Build history of the part. All positions in model axes, mm. Face numbers are marked on the shaded views. Give positions to 0.01 mm unless a question says otherwise; leave off trailing zeros. Loops run counter-clockwise (first coordinate to the right, second up) from the corner with the lowest first, then second, coordinate; pieces in that order, holes last. Notation, with made-up numbers: M 54.25,19.25 L 77.25,19.25 A13 cw 77.25,31.25 Z; hole C 41.25,38.25 d7. An arc over 180 degrees is marked long. Answer as a JSON object with one key per item and string values. Group by question number.
1. Mould opens along X. For the marked faces 1, 2, 3 and 4 say: released by +X, released by -X, zero draft, split by the parting line, or undercut.
2. Slice it at A-A (x = 0). List the corners of the cut face in (y, z).
3. Drill centre lines: line 1 along Y through (x, z) = (0, 3.2); line 2 along Z through (x, y) = (-1, -2); line 3 along Z through (x, y) = (-12.25, 1.5). Where is each one in solid material? Low to high. Write a range as [from, to].
4. Slice it at B-B (z = 0.3). List the corners of the cut face in (x, y) (3 decimals), then the cut area to 3 significant figures.
5. Drop flat-ended pins along their axis: pin 1 Ø1.5 at (x, z) = (-10.5, 3.5) entering from -Y; pin 2 Ø2 at (y, z) = (2.5, 0.5) entering from -X; pin 3 Ø3 at (x, y) = (0, 0) entering from +Z; pin 4 Ø1.7 at (x, y) = (-6.5, -1) entering from +Z. Give the stop position or say it passes through.
6. Slice it at D-D (z = 2.25). List the corners of the cut face in (x, y) (3 decimals).
7. Slice it at C-C (y = 0). Give the number of separate pieces and of enclosed holes in the cut face, then the cut area to 3 significant figures.
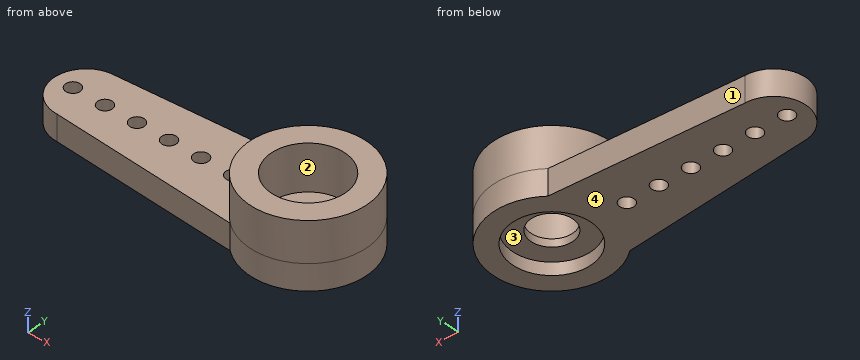
from build123d import *
from build123d.topology import SkipClean

# Parameters (mm, degrees)
RESSALTO_EXTRUS_O1_DEPTH = 1.6
ESBO_O2_R                = 3.65
RESSALTO_EXTRUS_O2_DEPTH = 2.5
ESBO_O3_R                = 2.3
CORTE_EXTRUS_O1_DEPTH    = 2.84
CORTE_EXTRUS_O2_REACH    = 18.456
ESBO_O4_R                = 0.45
ESBO_O5_R                = 1.3
CORTE_EXTRUS_O3_DEPTH    = 2.84
ESBO_O6_R                = 2.45
CORTE_EXTRUS_O4_DEPTH    = 0.78


with BuildPart() as part:
    # Esboço1 → Ressalto-extrusão1 (new body)
    with BuildSketch(Plane.XY):
        with BuildLine():
            Line((-13.85, 2), (-2.311249662, 2.825))
            ThreePointArc((-2.311249662, 2.825), (3.65, 0), (-2.311249662, -2.825))
            Line((-2.311249662, -2.825), (-13.85, -2))
            ThreePointArc((-13.85, -2), (-15.85, 0), (-13.85, 2))
        make_face()
    extrude(amount=RESSALTO_EXTRUS_O1_DEPTH)

    # Esboço2 → Ressalto-extrusão2 (add)
    with SkipClean():  # the faces are left unmerged after this step: merging them gives an invalid solid
        with BuildSketch(Plane.XY.offset(1.6)):
            with Locations(Location((0, 0, 0), (0, 0, 230.711977832))):
                Circle(ESBO_O2_R)
        extrude(amount=RESSALTO_EXTRUS_O2_DEPTH)

    # Esboço3 → Corte-extrusão1 (cut)
    with SkipClean():  # the faces are left unmerged after this step: merging them gives an invalid solid
        with BuildSketch(Plane.XY.offset(4.1)):
            Circle(ESBO_O3_R)
        extrude(amount=-CORTE_EXTRUS_O1_DEPTH, mode=Mode.SUBTRACT)

    # Esboço4 → Corte-extrusão2 (cut, up to next)
    with BuildSketch(Plane.XY.offset(1.6), mode=Mode.PRIVATE) as corte_extrus_o2_sk1:
        with Locations((-4.68, 0)):
            Circle(ESBO_O4_R)
    corte_extrus_o2_tool1 = extrude(corte_extrus_o2_sk1.sketch, amount=-CORTE_EXTRUS_O2_REACH, mode=Mode.PRIVATE) & part.part
    # Esboço4 → Corte-extrusão2 (cut, up to next)
    with BuildSketch(Plane.XY.offset(1.6), mode=Mode.PRIVATE) as corte_extrus_o2_sk2:
        with Locations((-6.68, 0)):
            Circle(ESBO_O4_R)
    corte_extrus_o2_tool2 = extrude(corte_extrus_o2_sk2.sketch, amount=-CORTE_EXTRUS_O2_REACH, mode=Mode.PRIVATE) & part.part
    # Esboço4 → Corte-extrusão2 (cut, up to next)
    with BuildSketch(Plane.XY.offset(1.6), mode=Mode.PRIVATE) as corte_extrus_o2_sk3:
        with Locations((-8.68, 0)):
            Circle(ESBO_O4_R)
    corte_extrus_o2_tool3 = extrude(corte_extrus_o2_sk3.sketch, amount=-CORTE_EXTRUS_O2_REACH, mode=Mode.PRIVATE) & part.part
    # Esboço4 → Corte-extrusão2 (cut, up to next)
    with BuildSketch(Plane.XY.offset(1.6), mode=Mode.PRIVATE) as corte_extrus_o2_sk4:
        with Locations((-10.68, 0)):
            Circle(ESBO_O4_R)
    corte_extrus_o2_tool4 = extrude(corte_extrus_o2_sk4.sketch, amount=-CORTE_EXTRUS_O2_REACH, mode=Mode.PRIVATE) & part.part
    # Esboço4 → Corte-extrusão2 (cut, up to next)
    with BuildSketch(Plane.XY.offset(1.6), mode=Mode.PRIVATE) as corte_extrus_o2_sk5:
        with Locations((-12.68, 0)):
            Circle(ESBO_O4_R)
    corte_extrus_o2_tool5 = extrude(corte_extrus_o2_sk5.sketch, amount=-CORTE_EXTRUS_O2_REACH, mode=Mode.PRIVATE) & part.part
    # Esboço4 → Corte-extrusão2 (cut, up to next)
    with BuildSketch(Plane.XY.offset(1.6), mode=Mode.PRIVATE) as corte_extrus_o2_sk6:
        with Locations((-14.68, 0)):
            Circle(ESBO_O4_R)
    corte_extrus_o2_tool6 = extrude(corte_extrus_o2_sk6.sketch, amount=-CORTE_EXTRUS_O2_REACH, mode=Mode.PRIVATE) & part.part
    add(corte_extrus_o2_tool1.solids().sort_by_distance((-4.68, 0, 1.6))[0], mode=Mode.SUBTRACT)
    add(corte_extrus_o2_tool2.solids().sort_by_distance((-6.68, 0, 1.6))[0], mode=Mode.SUBTRACT)
    add(corte_extrus_o2_tool3.solids().sort_by_distance((-8.68, 0, 1.6))[0], mode=Mode.SUBTRACT)
    add(corte_extrus_o2_tool4.solids().sort_by_distance((-10.68, 0, 1.6))[0], mode=Mode.SUBTRACT)
    add(corte_extrus_o2_tool5.solids().sort_by_distance((-12.68, 0, 1.6))[0], mode=Mode.SUBTRACT)
    add(corte_extrus_o2_tool6.solids().sort_by_distance((-14.68, 0, 1.6))[0], mode=Mode.SUBTRACT)

    # Esboço5 → Corte-extrusão3 (cut)
    with SkipClean():  # the faces are left unmerged after this step: merging them gives an invalid solid
        with BuildSketch(Plane(origin=(0, 0, 0), x_dir=(-1, 0, 0), z_dir=(0, 0, -1))):
            Circle(ESBO_O5_R)
        extrude(amount=-CORTE_EXTRUS_O3_DEPTH, mode=Mode.SUBTRACT)

    # Esboço6 → Corte-extrusão4 (cut)
    with SkipClean():  # the faces are left unmerged after this step: merging them gives an invalid solid
        with BuildSketch(Plane(origin=(0, 0, 0), x_dir=(-1, 0, 0), z_dir=(0, 0, -1))):
            Circle(ESBO_O6_R)
        extrude(amount=-CORTE_EXTRUS_O4_DEPTH, mode=Mode.SUBTRACT)


solid = part.part
Established:
{
 "1": {"face 1": "released by -X", "face 2": "undercut", "face 3": "undercut", "face 4": "zero draft"},
 "2": {"outline": "M -3.65,0 L -2.45,0 L -2.45,0.78 L -1.3,0.78 L -1.3,1.26 L -2.3,1.26 L -2.3,4.1 L -3.65,4.1 Z; M 1.3,0.78 L 2.45,0.78 L 2.45,0 L 3.65,0 L 3.65,4.1 L 2.3,4.1 L 2.3,1.26 L 1.3,1.26 Z"},
 "3": {"line 1": "y = [-3.65, -2.3], [2.3, 3.65]", "line 2": "z = [0.78, 1.26]", "line 3": "z = [0, 1.6]"},
 "4": {"outline": "M -13.85,-2 L -2.311,-2.825 A3.65 ccw long -2.311,2.825 L -13.85,2 A2 ccw Z; hole C -14.68,0 d0.9; hole C -12.68,0 d0.9; hole C -10.68,0 d0.9; hole C -8.68,0 d0.9; hole C -6.68,0 d0.9; hole C -4.68,0 d0.9; hole C 0,0 d4.9", "area": "75.9 mm^2"},
 "5": {"pin 1": "passes through", "pin 2": "stops at x = -15.17", "pin 3": "stops at z = 1.26", "pin 4": "stops at z = 1.6"},
 "6": {"outline": "C 0,0 d7.3; hole C 0,0 d4.6"},
 "7": {"separate pieces": "8", "enclosed holes": "0", "area": "22.7 mm^2"}
}
